The listing builds one solid part. Answer for the finished solid, in the listing's coordinates (mm). A direction names the side the tool comes from. Round coordinates to 2 decimals unless told otherwise and drop trailing zeros. Order: outer loops, then holes, each group sorted by start corner. A loop starts at its lowest first (then second) coordinate and runs counter-clockwise, first axis right, second up. Notation, with made-up numbers: (15.25, -35) - (20.25, -35) arc R14 cw to (20.25, -26) - close; hole circle Ø9 at (-32, -35.5). An arc over 180 degrees is marked (long way). One line per item, written item: value. Start each with the question number.
1. Section D-D, the plane x = 40 is taken. Give the vertices of the cut face in (y, z), then the cut area to 3 significant figures.
2. Section C-C, the plane y = -58.5 is taken. Give the vertices of the cut face in (x, z), then the cut area to 3 significant figures.
3. Section A-A, the plane z = 0.8 is taken. Give the vertices of the cut face in (x, y).
4. A tool of negligible diameter and unlimited length cuts with its end or side. For faces 4 (the flat face through (32, 53.71, 1.23)), 5 (the flat face through (77, -7, 5)), 6 (the flat face through (55, -80, 2.5)), from which of +Z, -Z, +X, -X, +Y, -Y can it reach the whole face along a straight path? Write none if from no direction.
5. Straight lines are drawn through the part: line 1 (Y direction, x = 54, z = 4.35); line 2 (Y direction, x = 70.5, z = 3.6); line 3 (Y direction, x = 66, z = 3.85). For each, find the intervals that lie inside material, in ascending order.
6. Flat-ended cylindrical pins translate along their axes: P1, Ø2, axis at y = 17.5, z = 1, coming from the -X side; P2, Ø2, axis at x = 30, y = 53, coming from the -Z side; P3, Ø5, axis at x = 53.19, y = -81.74, coming from the +Z side; P4, Ø1, axis at y = 30, z = 4, coming from the +X side. Find the tip coordinate at first contact, or state that the pin passes through.
7. Section B-B, the plane x = 66 is taken. Give the vertices of the cut face in (y, z), then the cut area to 3 significant figures.
8. For a pull along X with two mould halves and no side action, classify faces 1 (the flat face through (29, 55, 2.5)), 2 (the cylindrical face through (52.003, -82.65, 3.732)), 3 (the cylindrical face through (25.156, 56.779, 3.732)) as released by +X, released by -X, zero draft, split by the parting line, or undercut.
from build123d import *

# Parameters (mm, degrees)
F0_R     = 1.5
F1_DEPTH = 5
F2_DEPTH = 2.5
F4_DEPTH = 2.5


# Not quite as in the source:
# - a feature names something its author has since deleted; it is built from what else it names


with BuildPart() as f1:
    # F0 (on Top) → F1 (new body)
    with BuildSketch(Plane.XY):
        with BuildLine():
            Line((30, 51.9615242271), (32.4836596815, 56.2633489842))
            Line((32.4836596815, 56.2633489842), (28.4224519805, 58.0264243292))
            ThreePointArc((28.4224519805, 58.0264243292), (25.1336779708, 56.7287473614), (26.4313549386, 53.4399733516))
            Line((26.4313549386, 53.4399733516), (29.967319363, 51.9049197034))
            Line((29.967319363, 51.9049197034), (30, 51.9615242271))
        make_face()
        with Locations((27.4269034596, 55.7331988404)):
            Circle(F0_R, mode=Mode.SUBTRACT)
        with BuildLine():
            ThreePointArc((67.5061883913, 18.5179515304), (63.7494272333, 28.9138466382), (58.4029909795, 38.5887372772))
            ThreePointArc((58.4029909795, 38.5887372772), (46.511709986, 48.4848469682), (33.0089029581, 56.0353272873))
            Line((33.0089029581, 56.0353272873), (31.0178059162, 51.4488763097))
            ThreePointArc((31.0178059162, 51.4488763097), (51.8847287198, 37.8894735935), (67.5061883913, 18.5179515304))
        make_face()
        Polygon((31.0178059162, 51.4488763097), (33.0089029581, 56.0353272873), (32.4836596815, 56.2633489842), (30, 51.9615242271), (29.967319363, 51.9049197034), align=None)
        with BuildLine():
            ThreePointArc((54.2641944404, -83.9964118384), (54.5449950566, -83.8143395504), (54.8251847727, -83.6313285476))
            ThreePointArc((54.8251847727, -83.6313285476), (56.7197095597, -81.8911804241), (58.5601267726, -80.0939035554))
            Line((58.5601267726, -80.0939035554), (55.0705599201, -76.5129397591))
            ThreePointArc((55.0705599201, -76.5129397591), (53.341493873, -78.2050105238), (51.5614910891, -79.8434130866))
            ThreePointArc((51.5614910891, -79.8434130866), (51.0979794421, -83.1009956935), (54.2641944404, -83.9964118384))
        make_face()
        with Locations((53.1933379309, -81.7373708171)):
            Circle(F0_R, mode=Mode.SUBTRACT)
        with BuildLine():
            Line((55.0705599201, -76.5129397591), (58.5601267726, -80.0939035554))
            ThreePointArc((58.5601267726, -80.0939035554), (80.0342840094, -42.9250014233), (80.3674019431, 0))
            Line((80.3674019431, 0), (75.1959644791, 0))
            ThreePointArc((75.1959644791, 0), (75.3863719236, -40.9533729371), (55.0705599201, -76.5129397591))
        make_face()
        with BuildLine():
            ThreePointArc((54.2641944404, -83.9964118384), (54.5569628073, -83.8327293059), (54.8251847727, -83.6313285476))
            ThreePointArc((54.8251847727, -83.6313285476), (54.5449950566, -83.8143395504), (54.2641944404, -83.9964118384))
        make_face()
        with BuildLine():
            Line((75.1959644791, 0), (80.3674019431, 0))
            ThreePointArc((80.3674019431, 0), (71.977896021, 20.7701131861), (58.4029909795, 38.5887372772))
            ThreePointArc((58.4029909795, 38.5887372772), (63.7494272333, 28.9138466382), (67.5061883913, 18.5179515304))
            ThreePointArc((67.5061883913, 18.5179515304), (71.9402181457, 9.5036231189), (75.1959644791, 0))
        make_face()
    extrude(amount=F1_DEPTH)


with BuildPart() as f2:
    # F0 (on Top) → F2 (new body)
    with BuildSketch(Plane.XY):
        Polygon((31.0178059162, 51.4488763097), (33.0089029581, 56.0353272873), (32.4836596815, 56.2633489842), (30, 51.9615242271), (29.967319363, 51.9049197034), align=None)
        with BuildLine():
            Line((30, 51.9615242271), (32.4836596815, 56.2633489842))
            Line((32.4836596815, 56.2633489842), (28.4224519805, 58.0264243292))
            ThreePointArc((28.4224519805, 58.0264243292), (25.1336779708, 56.7287473614), (26.4313549386, 53.4399733516))
            Line((26.4313549386, 53.4399733516), (29.967319363, 51.9049197034))
            Line((29.967319363, 51.9049197034), (30, 51.9615242271))
        make_face()
        with Locations((27.4269034596, 55.7331988404)):
            Circle(F0_R, mode=Mode.SUBTRACT)
    extrude(amount=F2_DEPTH)


with BuildPart() as f1_1:
    add(f1.part)

    # F3: cut F2
    add(f2.part, mode=Mode.SUBTRACT)


with BuildPart() as f4:
    # F0 (on Top) → F4 (new body)
    with BuildSketch(Plane.XY):
        with BuildLine():
            ThreePointArc((54.2641944404, -83.9964118384), (54.5449950566, -83.8143395504), (54.8251847727, -83.6313285476))
            ThreePointArc((54.8251847727, -83.6313285476), (56.7197095597, -81.8911804241), (58.5601267726, -80.0939035554))
            Line((58.5601267726, -80.0939035554), (55.0705599201, -76.5129397591))
            ThreePointArc((55.0705599201, -76.5129397591), (53.341493873, -78.2050105238), (51.5614910891, -79.8434130866))
            ThreePointArc((51.5614910891, -79.8434130866), (51.0979794421, -83.1009956935), (54.2641944404, -83.9964118384))
        make_face()
        with Locations((53.1933379309, -81.7373708171)):
            Circle(F0_R, mode=Mode.SUBTRACT)
        with BuildLine():
            ThreePointArc((54.2641944404, -83.9964118384), (54.5569628073, -83.8327293059), (54.8251847727, -83.6313285476))
            ThreePointArc((54.8251847727, -83.6313285476), (54.5449950566, -83.8143395504), (54.2641944404, -83.9964118384))
        make_face()
    extrude(amount=F4_DEPTH)


with BuildPart() as f1_2:
    add(f1_1.part)

    # F5: cut F4
    add(f4.part, mode=Mode.SUBTRACT)


solid = f1_2.part
Answer list:
1. outline: (46.75, 0) - (52.53, 0) - (52.53, 5) - (46.75, 5) - close
1. area: 28.9 mm²
2. outline: (68.44, 0) - (74.08, 0) - (74.08, 5) - (68.44, 5) - close
2. area: 28.2 mm²
3. outline: (31.02, 51.45) arc R79.1 cw to (55.07, -76.51) - (58.56, -80.09) arc R84.1 ccw to (33.01, 56.04) - close
4. face 4: -Z, -X, +Y
4. face 5: +Z, +X, -X, +Y, -Y
4. face 6: -Z, -X, -Y
5. line 1: y = -84.1 to -83, -80.47 to -77.57, 35.91 to 42.69
5. line 2: y = -64.93 to -54.43, 12.76 to 23.27
5. line 3: y = -71.51 to -62.7, 21.04 to 29.85
6. P1: stops at x = 67.52
6. P2: stops at z = 2.5
6. P3: stops at z = 5
6. P4: stops at x = 66.26
7. outline: (-71.51, 0) - (-62.7, 0) - (-62.7, 5) - (-71.51, 5) - close; (21.04, 0) - (29.85, 0) - (29.85, 5) - (21.04, 5) - close
7. area: 88.2 mm²
8. face 1: zero draft
8. face 2: undercut
8. face 3: split by the parting line
